The listing builds one solid part. Answer for the finished solid, in the listing's coordinates (mm). Face numbers are marked on the shaded views. A direction names the side the tool comes from. Coordinates: 2 decimals unless noted, no trailing zeros. Loops run counter-clockwise (first coordinate to the right, second up) from the corner with the lowest first, then second, coordinate; pieces in that order, holes last. Notation, with made-up numbers: M -39,-37.75 L -30,-37.75 A32 ccw -30,-1.75 Z; hole C -25,58.5 d10. An arc over 180 degrees is marked long. Answer in a Markdown table with one row per item. Add a question column.
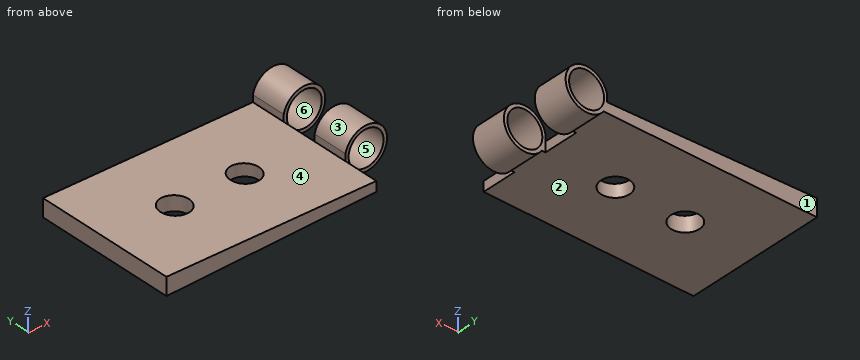
Autodesk Inventor part; units mm, degrees
ref_plane "Work Plane1" through (0, 12.7, 0) normal (0, -1, 0) x (1, 0, 0)
ref_plane "YZ Plane" through (0, 0, 0) normal (1, 0, 0) x (0, 1, 0)
ref_plane "XZ Plane" through (0, 0, 0) normal (0, 1, 0) x (-1, 0, 0)
sketch "Sketch1" plane through (0, 0, 0) normal (0, 0, 1) x (1, 0, 0)
  line L0 (0, 0) -> (38.1, 0)
  line L1 (38.1, 0) -> (38.1, 25.4)
  line L2 (38.1, 25.4) -> (0, 25.4)
  line L3 (0, 25.4) -> (0, 0)
  line L4 (0, 12.7) -> (12.7, 12.7) construction
  line L5 (12.7, 12.7) -> (25.4, 12.7) construction
  circle A0 centre (12.7, 12.7) radius 2.5797
  circle A1 centre (25.4, 12.7) radius 2.5797
  dimension "d0" = 38.1
  dimension "d1" = 25.4
  dimension "d2" = 12.7
  dimension "d3" = 12.7
  dimension "d4" = 5.1594
  dimension "d5" = 5.1594
extrude "Extrusion1" add sketch "Sketch1" along normal blind 3.175
sketch "Sketch2" plane through (0, 25.4, 0) normal (0, 1, 0) x (1, 0, 0)
  circle A0 centre (41.8269, -2.2431) radius 3.175
  arc A1 (38.1, -3.0347) -> (38.7472, 0) centre (41.8269, -2.2431) ccw
  line L0 (0, 0) -> (38.1, 0)
  line L1 (38.7472, 0) -> (38.1, 0)
  line L2 (38.1, 0) -> (38.1, -3.175)
  line L3 (38.1, 0) -> (38.1, -3.175)
  dimension "d8" = 6.35
  dimension "d9" = 7.62
extrude "Extrusion2" add sketch "Sketch2" against normal blind 6.35
ref_plane "Work Plane1" through (0, 12.7, 0) normal (0, -1, 0) x (1, 0, 0)
sketch "Sketch3" plane through (0, 12.7, 0) normal (0, -1, 0) x (1, 0, 0)
  arc A0 (38.7472, 0) -> (38.1, 3.0347) centre (41.8269, 2.2431) ccw
  circle A1 centre (41.8269, 2.2431) radius 3.175
  line L0 (38.1, 0) -> (38.7472, 0)
  line L1 (38.1, 0) -> (38.1, 3.0347)
  line L2 (38.1, 3.0347) -> (38.1, 0)
  point P0 (0, 0)
extrude "Extrusion3" add sketch "Sketch3" along normal blind 6.35
sketch "Sketch4" plane through (0, 25.4, 3.175) normal (0, 1, 0) x (1, 0, 0)
  line L0 (38.1, 0) -> (38.1, 1.3774)
  line L1 (0, 3.175) -> (0, 0)
  line L2 (38.1, 1.3774) -> (0, 0)
  line L3 (0, 0) -> (38.1, 0)
extrude "Extrusion4" cut sketch "Sketch4" against normal blind 50.8
properties part number "hinge"
(1) Each of these flat-tipped pins is pushed along its axis until it touches: pin 1 (0.5 mm diameter, centred on y = 15.5, z = 1.5, fed in from +X); pin 2 (2 mm diameter, centred on y = 6, z = 1.5, fed in from -X); pin 3 (5 mm diameter, centred on x = 10.5, y = 9.5, fed in from +Z); pin 4 (3 mm diameter, centred on x = 30, y = 10.5, fed in from +Z). Where does it stop, or does it pass through?
(2) Straight lines are drawn through the part: line 1 (Z direction, x = 42, y = 12.5); line 2 (Y direction, x = 12.7, z = 1.95); line 3 (X direction, y = 24.25, z = 4.5). For each, find the intervals that lie inside material, in ascending order.
(3) For the marked faces 1 and 2, determine the directions among +Z, -Z, +X, -X, +Y, -Y from which every point of the face is accessible in a straight line to the end or side of a thin tool.
(4) A cutting plane is placed at A-A (x = 12.7). Give the vertices of the cut face in (y, z), plus the area to 3 significant figures.
(5) A cutting plane is placed at D-D (y = 20). Give the vertices of the cut face in (x, z) (3 decimals).
(6) A cutting plane is placed at B-B (y = 10.75). Give the vertices of the cut face in (x, z) (3 decimals), plus the area to 3 significant figures.
(7) A cutting plane is placed at C-C (y = 13.5). Give the vertices of the cut face in (x, z) (3 decimals), plus the area to 3 significant figures.
(8) The mould has two halves that part along Z. Classify the marked faces 3, 4, 5 and 6: released by +Z, released by -Z, zero draft, split by the parting line, or undercut.
Solved:
| question | item | result |
|---|---|---|
| 1 | pin 1 | stops at x = 38.1 |
| 1 | pin 2 | stops at x = 0 |
| 1 | pin 3 | stops at z = 2.89 |
| 1 | pin 4 | stops at z = 2.14 |
| 2 | line 1 | z = -1.56 to -0.93, 5.41 to 6.05 |
| 2 | line 2 | y = 0 to 10.12, 15.28 to 25.4 |
| 2 | line 3 | x = 38.76 to 39.59, 44.06 to 44.9 |
| 3 | face 1 | +Z, -Z, +X, -X, +Y |
| 3 | face 2 | -Z, -X, +Y, -Y |
| 4 | outline | M 0,0 L 10.12,0 L 10.12,2.72 L 0,2.72 Z; M 15.28,0 L 25.4,0 L 25.4,2.72 L 15.28,2.72 Z |
| 4 | area | 55.0 mm² |
| 5 | outline | M 0,0 L 38.747,0 A3.81 ccw long 38.1,3.035 L 38.1,1.798 L 0,3.175 Z; hole C 41.827,2.243 d6.35 |
| 6 | outline | M 0,0 L 11.011,0 L 11.011,2.777 L 0,3.175 Z; M 14.389,0 L 23.711,0 L 23.711,2.318 L 14.389,2.655 Z; M 27.089,0 L 38.747,0 A3.81 ccw long 38.1,3.035 L 38.1,1.798 L 27.089,2.196 Z; hole C 41.827,2.243 d6.35 |
| 6 | area | 92.2 mm² |
| 7 | outline | M 0,0 L 10.247,0 L 10.247,2.805 L 0,3.175 Z; M 15.153,0 L 22.947,0 L 22.947,2.345 L 15.153,2.627 Z; M 27.853,0 L 38.1,0 L 38.1,1.798 L 27.853,2.168 Z |
| 7 | area | 70.3 mm² |
| 8 | face 3 | split by the parting line |
| 8 | face 4 | released by +Z |
| 8 | face 5 | undercut |
| 8 | face 6 | undercut |
